Work out the finished part from the listing and answer in its coordinate system (mm). A direction names the side the tool comes from. Give positions to 0.01 mm unless a question says otherwise; leave off trailing zeros. Loops run counter-clockwise (first coordinate to the right, second up) from the corner with the lowest first, then second, coordinate; pieces in that order, holes last. Notation, with made-up numbers: M -14.75,85.25 L 29.25,85.25 A20 cw 29.25,122.25 Z; hole C 59,86.5 d1. An arc over 180 degrees is marked long. Write item = value, one per line. Start each with the question number.
1. Flat-ended cylindrical pins translate along their axes: pin 1 Ø2 at (x, y) = (5.5, 0) entering from -Z; pin 2 Ø9.5 at (x, z) = (18, 6.5) entering from +Y; pin 3 Ø8 at (x, y) = (29.5, 7.5) entering from +Z. Find the tip coordinate at first contact, or state that the pin passes through.
2. For faces 1 (the face through (22, -8.5, -29)), 2 (the face through (8.81, 5.45, -43.22)), 3 (the face through (15.283, 28.696, -27.211)), determine the directions among +Z, -Z, +X, -X, +Y, -Y from which every point of the face is accessible in a straight line to the end or side of a thin tool.
3. Section C-C on x = 37 is taken. Give the number of separate pieces and of enclosed holes in the cut face, plus the area to 3 significant figures.
4. Consider L1, parallel to Z at x = 12, y = -5; L2, parallel to Y at x = 34.75, z = 15.5; L3, parallel to Z at x = 2.5, y = 6. Determine where each line is inside the solid, lowest interval first. Write a range as [from, to].
5. The mould has two halves that part along Z. Classify faces 4 (the face through (15.283, -19.696, -23.789)), 5 (the face through (22.185, -26.711, -98.696)), 6 (the face through (22, -40, -1)), 7 (the face through (4, -30, -88)): released by +Z, released by -Z, zero draft, split by the parting line, or undercut.
6. Section A-A on z = -88 is taken. Determine the outline of the cut face in (x, y), plus the area to 3 significant figures.
7. Section B-B on z = 0 is taken. Determine the outline of the cut face in (x, y).
Autodesk Inventor part; units mm, degrees
ref_plane "YZ Plane" through (0, 0, 0) normal (1, 0, 0) x (0, 1, 0)
ref_plane "XZ Plane" through (0, 0, 0) normal (0, 1, 0) x (-1, 0, 0)
ref_plane "XY Plane" through (0, 0, 0) normal (0, 0, 1) x (1, 0, 0)
sketch "Szkic1" plane through (0, 0, 0) normal (1, 0, 0) x (0, 1, 0)
  circle A0 centre (0, 0) radius 14
  arc A1 (15.7574, 63.5) -> (15.0197, 62.3339) centre (20, 60) ccw construction
  arc A2 (-20.25, 65.4943) -> (-15.0197, 62.3339) centre (-20, 60) ccw
  line L0 (20.25, 69.5) -> (-20.25, 69.5)
  line L1 (-20.25, 69.5) -> (-20.25, 65.4943)
  line L2 (-20.25, 63.5) -> (-15.7574, 63.5) construction
  line L3 (20.25, 63.5) -> (20.25, 65.4943) construction
  line L4 (15.7574, 63.5) -> (20.25, 63.5) construction
  line L5 (20.25, 65.4943) -> (20.25, 69.5)
  line L6 (-20.25, 65.4943) -> (-20.25, 63.5) construction
  line L7 (-15.7574, 63.5) -> (-13, 63.5) construction
  arc A3 (20.25, 65.4943) -> (15.7574, 63.5) centre (20, 60) ccw construction
  arc A4 (-15.7574, 63.5) -> (-20.25, 65.4943) centre (-20, 60) ccw construction
  line L8 (-15.0197, 62.3339) -> (-13, 63.5)
  line L9 (13, 63.5) -> (15.0197, 62.3339)
  arc A5 (15.0197, 62.3339) -> (20.25, 65.4943) centre (20, 60) ccw
  line L10 (13, 63.5) -> (15.7574, 63.5) construction
  arc A6 (-15.0197, 62.3339) -> (-15.7574, 63.5) centre (-20, 60) ccw construction
  line L11 (-13, 63.5) -> (13, 63.5)
  line L12 (14, 0) -> (-14, 0) construction
  arc A7 (15.0197, -62.3339) -> (15.7574, -63.5) centre (20, -60) ccw construction
  arc A8 (-15.0197, -62.3339) -> (-20.25, -65.4943) centre (-20, -60) ccw
  line L13 (20.25, -69.5) -> (-20.25, -69.5)
  line L14 (-20.25, -69.5) -> (-20.25, -65.4943)
  line L15 (-20.25, -63.5) -> (-15.7574, -63.5) construction
  line L16 (20.25, -63.5) -> (20.25, -65.4943) construction
  line L17 (15.7574, -63.5) -> (20.25, -63.5) construction
  line L18 (20.25, -65.4943) -> (20.25, -69.5)
  line L19 (-20.25, -65.4943) -> (-20.25, -63.5) construction
  line L20 (-15.7574, -63.5) -> (-13, -63.5) construction
  arc A9 (15.7574, -63.5) -> (20.25, -65.4943) centre (20, -60) ccw construction
  arc A10 (-20.25, -65.4943) -> (-15.7574, -63.5) centre (-20, -60) ccw construction
  line L21 (-15.0197, -62.3339) -> (-13, -63.5)
  line L22 (13, -63.5) -> (15.0197, -62.3339)
  arc A11 (20.25, -65.4943) -> (15.0197, -62.3339) centre (20, -60) ccw
  line L23 (13, -63.5) -> (15.7574, -63.5) construction
  arc A12 (-15.7574, -63.5) -> (-15.0197, -62.3339) centre (-20, -60) ccw construction
  line L24 (-13, -63.5) -> (13, -63.5)
  line L25 (24.5, 75.5) -> (-19, 75.5)
  line L26 (-40, 75.5) -> (-40, -75.5)
  line L27 (-19, -75.5) -> (24.5, -75.5)
  line L28 (30.5, -69.5) -> (30.5, -31.5)
  arc A13 (30.5, 69.5) -> (24.5, 75.5) centre (24.5, 69.5) ccw
  arc A14 (24.5, -75.5) -> (30.5, -69.5) centre (24.5, -69.5) ccw
  line L29 (-40, 75.5) -> (-25, 75.5) construction
  line L30 (-25, 81.5) -> (-25, 94.5)
  line L31 (-31, 100.5) -> (-40, 100.5)
  line L32 (-40, 100.5) -> (-40, 75.5)
  arc A15 (-25, 94.5) -> (-31, 100.5) centre (-31, 94.5) ccw
  arc A16 (-25, 81.5) -> (-19, 75.5) centre (-19, 81.5) ccw
  line L33 (-40, -75.5) -> (-25, -75.5) construction
  line L34 (-25, -81.5) -> (-25, -94.5)
  line L35 (-31, -100.5) -> (-40, -100.5)
  line L36 (-40, -100.5) -> (-40, -75.5)
  arc A17 (-31, -100.5) -> (-25, -94.5) centre (-31, -94.5) ccw
  arc A18 (-19, -75.5) -> (-25, -81.5) centre (-19, -81.5) ccw
  circle A19 centre (15.5, 15.5) radius 1.75
  circle A20 centre (15.5, -15.5) radius 1.75
  circle A21 centre (-15.5, 15.5) radius 1.75
  circle A22 centre (-15.5, -15.5) radius 1.75
  line L37 (15.5, -15.5) -> (-15.5, 15.5) construction
  line L38 (15.5, 15.5) -> (-15.5, -15.5) construction
  circle A23 centre (15.5, 15.5) radius 3.5
  circle A24 centre (15.5, -15.5) radius 3.5
  circle A25 centre (-15.5, -15.5) radius 3.5
  circle A26 centre (-15.5, 15.5) radius 3.5
  line L39 (24.5, -25.5) -> (-15.5, -25.5)
  line L40 (-21.5, -19.5) -> (-21.5, 19.5)
  line L41 (-15.5, 25.5) -> (24.5, 25.5)
  line L42 (30.5, 25.5) -> (30.5, -25.5) construction
  arc A27 (30.5, -31.5) -> (24.5, -25.5) centre (24.5, -31.5) ccw
  arc A28 (-21.5, -19.5) -> (-15.5, -25.5) centre (-15.5, -19.5) ccw
  arc A29 (-15.5, 25.5) -> (-21.5, 19.5) centre (-15.5, 19.5) ccw
  line L43 (30.5, 31.5) -> (30.5, 69.5)
  arc A30 (24.5, 25.5) -> (30.5, 31.5) centre (24.5, 31.5) ccw
  line L44 (30.5, -31.5) -> (30.5, 31.5)
  point P0 (-25, 100.5)
  point P1 (-25, -100.5)
  dimension "d0" = 28
  dimension "d1" = 11
  dimension "d2" = 40
  dimension "d3" = 20
  dimension "d4" = 60
  dimension "d6" = 6
  dimension "d8" = 3.5
  dimension "d9" = 150
  dimension "d10" = 150
  dimension "d11" = 26
  dimension "d12" = 13
  dimension "d13" = 6
  dimension "d14" = 6
  dimension "d15" = 10.5
  dimension "d16" = 20
  dimension "d17" = 6
  dimension "d18" = 15
  dimension "d19" = 25
  dimension "d20" = 6
  dimension "d21" = 15
  dimension "d22" = 25
  dimension "d23" = 6
  dimension "d24" = 3.5
  dimension "d25" = 31
  dimension "d26" = 31
  dimension "d27" = 7
  dimension "d34" = 10
  dimension "d35" = 10
  dimension "d36" = 6
  dimension "d37" = 6
  dimension "d38" = 6
  dimension "d50" = 0.25
  dimension "d51" = 0.25
extrude "Wyciągnięcie proste1" add sketch "Szkic1" along normal blind 45 contours A0 | L1 L0 L5 A5 L9 L11 L8 A2 | L21 L24 L22 A11 L18 L13 L14 A8 | A13 L43 A30 L41 A29 L40 A28 L39 A27 L28 A14 L27 A18 L34 A17 L35 L36 L26 L32 L31 A15 L30 A16 L25 | L44 A27 L39 A28 L40 A29 L41 A30 | A19 | A20 | A21 | A22 | A23 | A24 | A25 | A26
extrude "Wyciągnięcie proste2" cut sketch "Szkic1" along normal blind 31 contours A0 | L44 A27 L39 A28 L40 A29 L41 A30 | A19 | A20 | A21 | A22 | A23 | A24 | A25 | A26
extrude "Wyciągnięcie proste12" cut sketch "Szkic1" along normal through all contours L1 L0 L5 A5 L9 L11 L8 A2 | L21 L24 L22 A11 L18 L13 L14 A8
extrude "Wyciągnięcie proste4" cut sketch "Szkic1" along normal through all contours A0 | A19 | A20 | A21 | A22
sketch "Szkic2" plane through (0, -25, 94.5) normal (0, 1, 0) x (1, 0, 0)
  circle A0 centre (37, 6.5) radius 5.5
  circle A1 centre (8, 6.5) radius 5.5
  circle A2 centre (37, 6.5) radius 3.25
  circle A3 centre (8, 6.5) radius 3.25
  line L0 (45, 13) -> (45, 0)
  line L1 (0, -6) -> (45, -6)
  line L2 (0, 13) -> (0, 0)
  point P0 (0, 94.5)
  dimension "d41" = 6.5
  dimension "d42" = 11
  dimension "d43" = 8
  dimension "d44" = 12.5
  dimension "d45" = 8
extrude "Wyciągnięcie proste5" cut sketch "Szkic2" against normal through all contours A2 | A3
extrude "Wyciągnięcie proste6" cut sketch "Szkic2" against normal blind 5
mirror "Odbij1" about plane through (0, 0, 0) normal (0, 0, 1) of "Wyciągnięcie proste6", "Wyciągnięcie proste5"
sketch "Szkic5" plane through (0, -15.5, -25.5) normal (0, 0, 1) x (1, 0, 0)
  circle A0 centre (8, 22.5) radius 1.75
  circle A1 centre (8, 12.5) radius 1.75
  line L0 (0, 0) -> (0, 40)
  line L1 (31, 46) -> (0, 46)
  line L2 (31, 46) -> (0, 46)
  line L3 (0, 46) -> (45, 46)
  line L4 (0, 46) -> (45, 46)
  point P0 (0, 15.5)
  dimension "d63" = 3.5
  dimension "d64" = 3.5
  dimension "d65" = 8
  dimension "d66" = 10
  dimension "d67" = 23.5
extrude "Wyciągnięcie proste8" cut sketch "Szkic5" against normal blind 20
sketch "Szkic3" plane through (0, 0, 0) normal (-1, 0, 0) x (0, 0, 1)
  line L0 (-25.5, -15.5) -> (-25.5, 24.5)
  line L1 (-25.5, 12.5) -> (-32, 12.5)
  line L2 (-32, 12.5) -> (-32, -8.5)
  line L3 (-32, -8.5) -> (-25.5, -8.5)
  line L4 (-25.5, -8.5) -> (-25.5, 12.5)
  line L5 (-69.5, 30.5) -> (-31.5, 30.5)
  line L6 (-41, 10) -> (-38.4, 10)
  line L7 (-38.4, 10) -> (-38.4, 4)
  line L8 (-38.4, 4) -> (-41, 4)
  line L9 (-41, 4) -> (-41, 10)
  line L10 (-41, 0) -> (-38.4, 0)
  line L11 (-38.4, 0) -> (-38.4, -6)
  line L12 (-38.4, -6) -> (-41, -6)
  line L13 (-41, -6) -> (-41, 0)
  point P0 (0, 0)
  dimension "d52" = 21
  dimension "d53" = 6.5
  dimension "d54" = 18
  dimension "d55" = 2.6
  dimension "d56" = 6
  dimension "d57" = 6
  dimension "d58" = 2.5
  dimension "d59" = 2.5
  dimension "d60" = 9
extrude "Wyciągnięcie proste7" cut sketch "Szkic3" against normal through all contours L3 L2 L1 L0
extrude "Wyciągnięcie proste9" cut sketch "Szkic3" against normal blind 11 contours L6 L7 L8 L9 | L10 L11 L12 L13
sketch "Szkic6" plane through (0, 30.5, 69.5) normal (0, 1, 0) x (1, 0, 0)
  line L0 (24, 106.5) -> (40, 106.5)
  line L1 (40, 106.5) -> (40, 112.3)
  line L2 (40, 112.3) -> (34, 112.3)
  line L3 (24, 112.3) -> (24, 106.5)
  line L4 (34, 112.3) -> (34, 114)
  line L5 (34, 114) -> (30, 114)
  line L6 (30, 114) -> (30, 112.3)
  line L7 (0, 101.5) -> (45, 101.5)
  line L8 (0, 101.5) -> (45, 101.5)
  line L9 (6.25, 101.5) -> (9.75, 101.5)
  line L10 (6.25, 101.5) -> (9.75, 101.5)
  line L11 (45, 139) -> (45, 0)
  line L12 (30, 112.3) -> (24, 112.3)
  line L13 (34, 112.3) -> (30, 112.3) construction
  point P0 (0, 69.5)
  dimension "d77" = 5.8
  dimension "d79" = 4
  dimension "d80" = 1.7
  dimension "d81" = 6
  dimension "d82" = 16
  dimension "d83" = 5
  dimension "d84" = 5
extrude "Wyciągnięcie proste10" cut sketch "Szkic6" against normal blind 30
sketch "Szkic7" plane through (45, 0, 0) normal (1, 0, 0) x (0, 0, -1)
  line L0 (42.8, 30.5) -> (37, 30.5)
  line L1 (42.8, 30.5) -> (42.8, 0.5)
  line L2 (42.8, 0.5) -> (37, 0.5)
  line L3 (37, 30.5) -> (37, 0.5)
  line L4 (42.8, 0.5) -> (37, 0.5)
  line L5 (42.8, 30.5) -> (42.8, 0.5)
  line L6 (37, 0.5) -> (42.8, 0.5)
  line L7 (42.8, 0.5) -> (42.8, 12.5)
  line L8 (42.8, 12.5) -> (37, 12.5)
  line L9 (37, 12.5) -> (37, 0.5)
  point P0 (0, 0)
  point P1 (37, 12.5)
  dimension "d87" = 12
extrude "Wyciągnięcie proste11" cut sketch "Szkic7" against normal up to next contours L1 L2 L3 L8
equation "\"d14\" = d13"
equation "\"d38\" = d37"
properties part number "XMotorMount" material "Tworzywo sztuczne ABS"
Verdict:
q1.pin_1 = -75.5
q1.pin_2 = -21.5
q1.pin_3 = 75.5
q2.face_1 = +X, -X
q2.face_2 = none
q2.face_3 = -X, +Y
q3.separate_pieces = 3
q3.enclosed_holes = 8
q3.area = 9,330 mm2
q4.L1 = [-75.5, -69.5], [-63.5, -32], [25.5, 63.5], [69.5, 75.5]
q4.L2 = [-40, -17.25], [-13.75, 13.75], [17.25, 30.5]
q4.L3 = [-75.5, -69.5], [-63.5, -41], [-38.4, -32], [25.5, 63.5], [69.5, 75.5]
q5.face_4 = undercut
q5.face_5 = released by -Z
q5.face_6 = zero draft
q5.face_7 = undercut
q6.outline = M 0,-40 L 4.75,-40 L 4.75,-30 L 2.5,-30 L 2.5,-25 L 0,-25 Z; M 11.25,-40 L 33.75,-40 L 33.75,-30 L 31.5,-30 L 31.5,-25 L 13.5,-25 L 13.5,-30 L 11.25,-30 Z; M 40.25,-40 L 45,-40 L 45,-25 L 42.5,-25 L 42.5,-30 L 40.25,-30 Z
q6.area = 435 mm2
q7.outline = M 0,-40 L 45,-40 L 45,-14 L 31,-14 L 31,-21.5 L 0,-21.5 Z; M 31,14 L 45,14 L 45,30.5 L 31,30.5 Z
